from build123d import *

# Parameters (mm, degrees)
SKETCH1_R                            = 5
SKETCH1_R_2                          = 3
BOSS_EXTRUDE1_DEPTH                  = 1
SKETCH1_3_R                          = 5
SKETCH1_3_R_2                        = 3
BOSS_EXTRUDE2_DEPTH                  = 4
CHAMFER1_SIZE                        = 0.25
SKETCH5_R                            = 6.35
BOSS_EXTRUDE4_DEPTH                  = 4.7625
F_3_5_3_5_DIAMETER_HOLE1_D           = 3.5
F_3_5_3_5_DIAMETER_HOLE1_DEPTH       = 4.451427784
F_3_5_3_5_DIAMETER_HOLE1_CSINK_D     = 4
F_3_5_3_5_DIAMETER_HOLE1_CSINK_ANGLE = 90
F_3_5_3_5_DIAMETER_HOLE1_TIP         = 0.308572216
CHAMFER2_SIZE                        = 0.25
CHAMFER3_SIZE                        = 0.5


with BuildPart() as part:
    # Sketch1 → Boss-Extrude1 (new body)
    with BuildSketch(Plane(origin=(0, 0, 0), x_dir=(1, 0, 0), z_dir=(0, 1, 0))):
        with Locations(Location((0, 0, 0), (0, 0, 270))):
            Circle(SKETCH1_R)
        Circle(SKETCH1_R_2, mode=Mode.SUBTRACT)
        Circle(SKETCH1_R_2)
    extrude(amount=BOSS_EXTRUDE1_DEPTH)

    # Sketch1_3 → Boss-Extrude2 (add)
    with BuildSketch(Plane(origin=(0, 0, 0), x_dir=(1, 0, 0), z_dir=(0, 1, 0))):
        with Locations(Location((0, 0, 0), (0, 0, 270))):
            Circle(SKETCH1_3_R)
        with Locations(Location((0, 0, 0), (0, 0, 270))):
            Circle(SKETCH1_3_R_2, mode=Mode.SUBTRACT)
    extrude(amount=BOSS_EXTRUDE2_DEPTH)

    # Chamfer1
    chamfer1_edges = [part.edges().sort_by_distance(p)[0] for p in [
        (0, 1, -3),
        (0, 4, -5),
        (0, 4, -3),
    ]]
    chamfer(chamfer1_edges, length=CHAMFER1_SIZE)

    # Sketch5 → Boss-Extrude4 (add)
    with BuildSketch(Plane(origin=(0, 0, 0), x_dir=(1, 0, 0), z_dir=(0, 1, 0))):
        with Locations(Location((0, 0, 0), (0, 0, 270))):
            Circle(SKETCH5_R)
    extrude(amount=-BOSS_EXTRUDE4_DEPTH)

    # 3.5 _3.5_ Diameter Hole1
    with Locations(Plane(origin=(0, -4.7625, 0), x_dir=(-1, 0, 0), z_dir=(0, -1, 0))):
        with Locations((0, 0)):
            CounterSinkHole(F_3_5_3_5_DIAMETER_HOLE1_D / 2, F_3_5_3_5_DIAMETER_HOLE1_CSINK_D / 2, depth=F_3_5_3_5_DIAMETER_HOLE1_DEPTH, counter_sink_angle=F_3_5_3_5_DIAMETER_HOLE1_CSINK_ANGLE)
            with Locations((0, 0, -(F_3_5_3_5_DIAMETER_HOLE1_DEPTH + F_3_5_3_5_DIAMETER_HOLE1_TIP / 2))):  # 160° drill point
                Cone(0, F_3_5_3_5_DIAMETER_HOLE1_D / 2, F_3_5_3_5_DIAMETER_HOLE1_TIP, mode=Mode.SUBTRACT)

    # Chamfer2
    chamfer2_edges = [part.edges().sort_by_distance(p)[0] for p in [
        (0, -4.7625, -6.35),
        (0, 0, -6.35),
    ]]
    chamfer(chamfer2_edges, length=CHAMFER2_SIZE)

    # Chamfer3
    chamfer3_edges = [part.edges().sort_by_distance(p)[0] for p in [
        (0, 0, -5),
    ]]
    chamfer(chamfer3_edges, length=CHAMFER3_SIZE)


solid = part.part
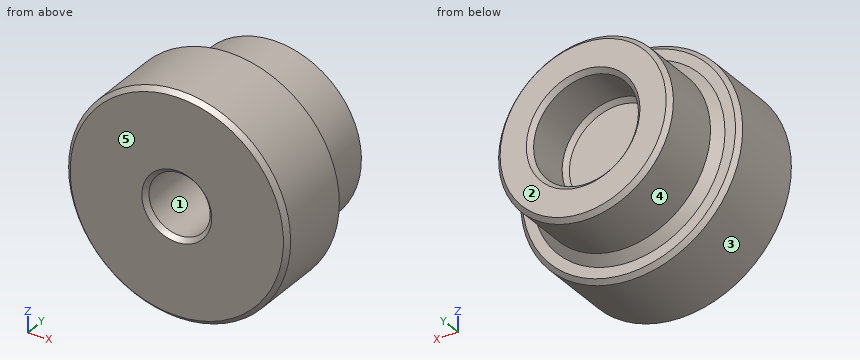
The model under review builds one solid part; all positions refer to its coordinate system, in mm. Face numbers are marked on the shaded views. A direction names the side the tool comes from. Give positions to 0.01 mm unless a question says otherwise; leave off trailing zeros. Write each loop counter-clockwise with the first axis right and the second up, starting at its lowest first coordinate (ties: lowest second). Pieces come first, ordered by that corner, then holes.
1. Add section A-A, the plane y = -2.5. Write out the cut boundary in (x, z), plus the area to 3 significant figures.
2. Add section B-B, the plane y = 0.25. Write out the cut boundary in (x, z), plus the area to 3 significant figures.
3. Wall thickness on L1, parallel to X at y = 2.45, z = 0; L2, parallel to Y at x = -3, z = -5; L3, parallel to X at y = 1.75, z = 2.25: over which ranges is each line inside the solid? List them lowest first.
4. Draft analysis for pull direction Z (two halves, no side actions). For the marked faces 1, 2 and 3, state which applies: +Z half, -Z half, draft (parallel to the pull), parting line (faces both ways), or undercut.
5. For P1, Ø1.5, axis at x = -3, y = 1.5, coming from the +Z side; P2, Ø3, axis at y = 0.5, z = -2, coming from the +X side, all flat-tipped, find the tip position at first contact; note any pin that passes through.
6. Tool access review of the marked faces 4 and 5: name each direction out of +Z, -Z, +X, -X, +Y, -Y from which nothing blocks a thin tool from reaching the whole face with its end or side.
Worked answers:
1. outline: circle Ø12.7 at (0, 0); hole circle Ø3.5 at (0, 0)
1. area: 117 mm2
2. outline: circle Ø10.5 at (0, 0)
2. area: 86.6 mm2
3. L1: x = -5 to -3, 3 to 5
3. L2: y = -4.76 to 0
3. L3: x = -4.47 to -1.98, 1.98 to 4.47
4. face 1: undercut
4. face 2: draft
4. face 3: parting line
5. P1: stops at z = 4.47
5. P2: stops at x = 6.31
6. face 4: +Y
6. face 5: +Z, -Z, +X, -X, -Y
